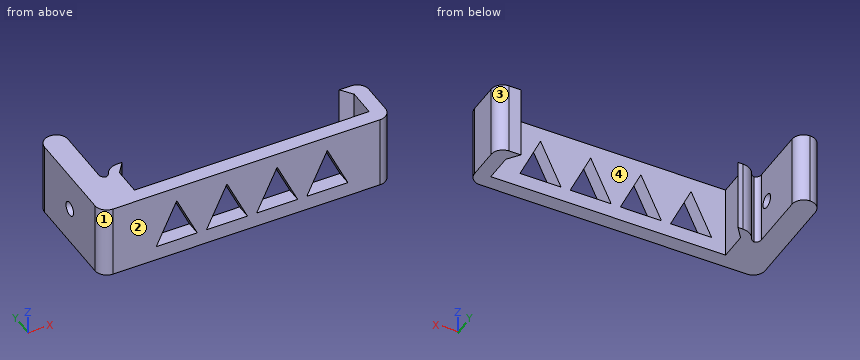
from build123d import *

# Parameters (mm, degrees)
F1_DEPTH    = 25
F2_T1_DEPTH = 25
F3_R        = 5
F4_R        = 3.99999
F5_R        = 2.4
F6_DEPTH    = 8
F8_DEPTH    = 5


# Not quite as in the source:
# - a fillet or chamfer that OpenCascade refuses, or shapes differently, is made with other operations: its cross-section is extruded or revolved along the edge and cut away or added
# - a fillet or chamfer is up to 0.001 mm smaller than in the source, because OpenCascade refuses the exact size


with BuildPart() as f1:
    # F0 (on Top) → F1 (new body)
    with BuildSketch(Plane.XY):
        Polygon((8, 40), (0, 40), (0, 0), (99, 0), (99, 18.5), (91, 18.5), (94, 14.5), (94, 5), (14, 5), (14, 14.5), (17, 18.5), (11, 18.5), (11, 14.5), (8, 14.5), align=None)
    extrude(amount=F1_DEPTH)

    # F2: fillet of radius 2 on 2 edges, made by hand

    # F2_s2 → F2_t1 (join)
    with BuildSketch(Plane.XY):
        with BuildLine():
            ThreePointArc((11, 16.5), (10.4142135624, 15.0857864376), (9, 14.5))
            Line((9, 14.5), (11, 14.5))
            Line((11, 14.5), (11, 16.5))
        make_face()
        with BuildLine():
            ThreePointArc((10, 14.5), (8.5857864376, 15.0857864376), (8, 16.5))
            Line((8, 16.5), (8, 14.5))
            Line((8, 14.5), (10, 14.5))
        make_face()
    extrude(amount=F2_T1_DEPTH)

    # F3
    f3_edges = [f1.edges().sort_by_distance(p)[0] for p in [
        (11, 18.5, 12.5),
    ]]
    fillet(f3_edges, radius=F3_R)

    # F4 (radius 4 in the source; OpenCascade refuses exactly that, so slightly less here)
    f4_edges = [f1.edges().sort_by_distance(p)[0] for p in [
        (99, 18.5, 12.5),
        (99, 0, 12.5),
        (0, 0, 12.5),
        (0, 40, 12.5),
        (8, 40, 12.5),
    ]]
    fillet(f4_edges, radius=F4_R)

    # F5 (on face) → F6 (cut, through all)
    with BuildSketch(Plane(origin=(0, 0, 0), x_dir=(0, -1, 0), z_dir=(-1, 0, 0))):
        with Locations((-20, 12.5)):
            Circle(F5_R)
    extrude(amount=-F6_DEPTH, mode=Mode.SUBTRACT)

    # F7 (on face) → F8 (cut, through all)
    with BuildSketch(Plane(origin=(0, 5, 0), x_dir=(-1, 0, 0), z_dir=(0, 1, 0))):
        Polygon((-77.0584673027, 20), (-84.053082175, 5), (-70.0638524304, 5), align=None)
        Polygon((-66.953082175, 5), (-52.9638524304, 5), (-59.9584673027, 20), align=None)
        Polygon((-49.853082175, 5), (-35.8638524304, 5), (-42.8584673027, 20), align=None)
        Polygon((-32.753082175, 5), (-18.7638524304, 5), (-25.7584673027, 20), align=None)
    extrude(amount=-F8_DEPTH, mode=Mode.SUBTRACT)


solid = f1.part
CAD build for the part. Positions are in the model's coordinates, mm. Face numbers are marked on the shaded views. Coordinates: 2 decimals unless noted, no trailing zeros. Order: outer loops, then holes, each group sorted by start corner. A loop starts at its lowest first (then second) coordinate and runs counter-clockwise, first axis right, second up. Notation, with made-up numbers: (49, 37) -> (54, 37) arc R29 ccw to (54, 59) -> close; hole circle Ø11 at (89, -14.75). An arc over 180 degrees is marked (long way). Answer in a Markdown table with one row per item.
1) Drill centre lines: line 1 (X direction, y = 14.5, z = 19.25); line 2 (Z direction, x = 3, y = 20); line 3 (Y direction, x = 92.5, z = 6.5). Where is each one in solid material? Low to high.
Check values:
| item | result |
|---|---|
| line 1 | 0 to 14, 94 to 99 |
| line 2 | 0 to 10.1, 14.9 to 25 |
| line 3 | 0 to 5, 16.5 to 18.5 |
2) Mould opens along X. For the marked faces 1, 2, 3 and 4 say: pulls with the +X half, pulls with the -X half, needs draft (parallel to the pull), parting line crosses it, or undercut.
Check values:
| item | result |
|---|---|
| face 1 | pulls with the -X half |
| face 2 | needs draft |
| face 3 | pulls with the +X half |
| face 4 | undercut |
3) Band-saw the part on C-C (z = 9). Give the number of separate pieces and of enclosed holes in the cut face, and give its area (3 significant figures).
Check values:
| item | result |
|---|---|
| separate pieces | 5 |
| enclosed holes | 0 |
| area | 700 mm2 |
4) Band-saw the part on B-B (x = 63.5). List the corners of the cut face in (y, z), and give its area (3 significant figures).
Check values:
| item | result |
|---|---|
| outline | (0, 0) -> (5, 0) -> (5, 5) -> (0, 5) -> close; (0, 12.41) -> (5, 12.41) -> (5, 25) -> (0, 25) -> close |
| area | 88.0 mm2 |
5) Flat gauge pins, fed straight in: P1, Ø4.5, axis at x = 92, z = 7.5, coming from the +Y side; P2, Ø6, axis at x = 49.5, y = 5.5, coming from the +Z side; P3, Ø4, axis at y = 28.5, z = 20, coming from the +X side; P4, Ø1, axis at x = 31.5, z = 18, coming from the +Y side. Where does each tip first touch, or does it go through?
Check values:
| item | result |
|---|---|
| P1 | y = 18.5 |
| P2 | z = 25 |
| P3 | x = 8 |
| P4 | y = 5 |
6) Band-saw the part on A-A (y = 20). List the corners of the cut face in (x, z).
Check values:
| item | result |
|---|---|
| outline | (0, 0) -> (8, 0) -> (8, 10.1) -> (0, 10.1) -> close; (0, 14.9) -> (8, 14.9) -> (8, 25) -> (0, 25) -> close |
7) Band-saw the part on D-D (y = 24.5). List the corners of the cut face in (x, z), and give its area (3 significant figures).
Check values:
| item | result |
|---|---|
| outline | (0, 0) -> (8, 0) -> (8, 25) -> (0, 25) -> close |
| area | 200 mm2 |
